Check sheet for the modelled part. Datum: model origin and axes. Units: mm. A direction names the side the tool comes from. Give positions to 0.01 mm unless a question says otherwise; leave off trailing zeros. Write each loop counter-clockwise with the first axis right and the second up, starting at its lowest first coordinate (ties: lowest second). Pieces come first, ordered by that corner, then holes. Notation, with made-up numbers: M 11,27 L 45,27 A25 ccw 45,58 Z; hole C 22.25,37 d8. An arc over 180 degrees is marked long. Write item = value, one per line. Start each with the question number.
1) Scan lines: L1, parallel to Y at x = 13.5, z = 0; L2, parallel to Y at x = 37.5, z = -59. Record each from-to range of solid material in increasing order.
2) Draft check along Z on faces 3 (the face through (1.97, 20.85, -32.11)), 4 (the face through (0, 0, 0)). Enter one of: pulls with the +Z half, pulls with the -Z half, needs draft (parallel to the pull), parting line crosses it, or undercut.
3) Gauge pin test, flat ends, axial feed: pin 1 (12 mm diameter, centred on x = 10, z = -8, fed in from -Y); pin 2 (10 mm diameter, centred on y = -2, z = 3.5, fed in from -X); pin 3 (2 mm diameter, centred on x = 6, y = 14, fed in from -Z); pin 4 (10 mm diameter, centred on y = -10, z = 39.5, fed in from +X). Record the tip position at first contact, or that the pin passes through.
4) Set-up check for faces 1 (the face through (1.97, 58.69, -33.34)), 2 (the face through (4, 0, 0)): record each of +Z, -Z, +X, -X, +Y, -Y from which the full face is reachable in a straight line by a thin tool's end or side.
5) Sectioned sample at C-C, the plane y = -43. Record the cut outline in (x, z), then the cut area to 3 significant figures.
6) Sectioned sample at D-D, the plane x = 34.5. Record the cut outline in (y, z), then the cut area to 3 significant figures.
7) Sectioned sample at B-B, the plane z = 48. Record the cut outline in (x, y).
8) Sectioned sample at A-A, the plane y = -22. Record the cut outline in (x, z).
Autodesk Inventor part; units mm, degrees
ref_plane "YZ Plane" through (0, 0, 0) normal (1, 0, 0) x (0, 1, 0)
ref_plane "XZ Plane" through (0, 0, 0) normal (0, 1, 0) x (-1, 0, 0)
ref_plane "XY Plane" through (0, 0, 0) normal (0, 0, 1) x (1, 0, 0)
sketch "Sketch1" plane through (0, 0, 0) normal (1, 0, 0) x (0, 1, 0)
  arc A0 (35.4672, -57.431) -> (67.4704, -2) centre (0, 0) ccw
  circle A1 centre (0, 0) radius 71.5
  arc A2 (3.1669, 9.4853) -> (-3.1669, 9.4853) centre (0, 0) ccw
  line L0 (10, 0) -> (67.5, 0) construction
  line L1 (9.798, 2) -> (67.4704, 2)
  line L2 (9.798, -2) -> (67.4704, -2)
  line L3 (3.1669, 9.4853) -> (32.0031, 59.431)
  line L4 (6.631, 7.4853) -> (35.4672, 57.431)
  line L5 (-6.631, 7.4853) -> (-35.4672, 57.431)
  line L6 (-3.1669, 9.4853) -> (-32.0031, 59.431)
  line L7 (-9.798, -2) -> (-67.4704, -2)
  line L8 (-9.798, 2) -> (-67.4704, 2)
  line L9 (-3.1669, -9.4853) -> (-32.0031, -59.431)
  line L10 (-6.631, -7.4853) -> (-35.4672, -57.431)
  line L11 (6.631, -7.4853) -> (35.4672, -57.431)
  line L12 (3.1669, -9.4853) -> (32.0031, -59.431)
  arc A3 (6.631, 7.4853) -> (3.1669, 9.4853) centre (0, 0) ccw
  arc A4 (-6.631, 7.4853) -> (-9.798, 2) centre (0, 0) ccw
  arc A5 (-3.1669, 9.4853) -> (-6.631, 7.4853) centre (0, 0) ccw
  arc A6 (-9.798, 2) -> (-9.798, -2) centre (0, 0) ccw
  arc A7 (-9.798, -2) -> (-6.631, -7.4853) centre (0, 0) ccw
  arc A8 (-6.631, -7.4853) -> (-3.1669, -9.4853) centre (0, 0) ccw
  arc A9 (-3.1669, -9.4853) -> (3.1669, -9.4853) centre (0, 0) ccw
  arc A10 (3.1669, -9.4853) -> (6.631, -7.4853) centre (0, 0) ccw
  arc A11 (6.631, -7.4853) -> (6.631, 7.4853) centre (0, 0) ccw
  arc A12 (32.0031, -59.431) -> (35.4672, -57.431) centre (0, 0) ccw
  arc A13 (67.4704, -2) -> (67.4704, 2) centre (0, 0) ccw construction
  arc A14 (35.4672, 57.431) -> (32.0031, 59.431) centre (0, 0) ccw construction
  arc A15 (32.0031, 59.431) -> (-32.0031, 59.431) centre (0, 0) ccw
  arc A16 (-32.0031, 59.431) -> (-35.4672, 57.431) centre (0, 0) ccw construction
  arc A17 (-35.4672, 57.431) -> (-67.4704, 2) centre (0, 0) ccw
  arc A18 (-67.4704, 2) -> (-67.4704, -2) centre (0, 0) ccw construction
  arc A19 (-67.4704, -2) -> (-35.4672, -57.431) centre (0, 0) ccw
  arc A20 (-35.4672, -57.431) -> (-32.0031, -59.431) centre (0, 0) ccw construction
  arc A21 (-32.0031, -59.431) -> (32.0031, -59.431) centre (0, 0) ccw
  arc A22 (67.4704, 2) -> (35.4672, 57.431) centre (0, 0) ccw
  dimension "d0" = 135
  dimension "d1" = 4
  dimension "d2" = 20
  dimension "d3" = 2
  dimension "d4" = 2
  dimension "d7" = 360
extrude "Extrusion1" add sketch "Sketch1" along normal blind 4 contours A12 L12 A10 L11 | A10 A9 A8 A7 A6 A4 A5 A2 A3 A11 | A1
sketch "Sketch2" plane through (4, 0, 0) normal (1, 0, 0) x (0, 0, -1)
  circle A0 centre (0, 0) radius 71.5
  line L0 (-59.431, 32.0031) -> (-9.4853, 3.1669)
  circle A1 centre (0, 0) radius 67.5
extrude "Extrusion2" add sketch "Sketch2" along normal blind 40
properties part number "SuportMotor"
Data:
q1.L1 = -71.5 to -67.5, 67.5 to 71.5
q1.L2 = -40.39 to -32.79, 32.79 to 40.39
q2.face_3 = undercut
q2.face_4 = needs draft
q3.pin_1 = -71.47
q3.pin_2 = 0
q3.pin_3 = -70.31
q3.pin_4 = through
q4.face_1 = +X, -X
q4.face_2 = +X
q5.outline = M 0,-57.12 L 44,-57.12 L 44,-52.03 L 0,-52.03 Z; M 0,-2 L 4,-2 L 4,2 L 0,2 Z; M 0,52.03 L 44,52.03 L 44,57.12 L 0,57.12 Z
q5.area = 464 mm2
q6.outline = C 0,0 d143; hole C 0,0 d135
q6.area = 1,750 mm2
q7.outline = M 0,-52.99 L 44,-52.99 L 44,-47.46 L 0,-47.46 Z; M 0,-30.02 L 4,-30.02 L 4,-25.4 L 0,-25.4 Z; M 0,25.4 L 4,25.4 L 4,30.02 L 0,30.02 Z; M 0,47.46 L 44,47.46 L 44,52.99 L 0,52.99 Z
q8.outline = M 0,-68.03 L 44,-68.03 L 44,-63.81 L 0,-63.81 Z; M 0,-42.11 L 4,-42.11 L 4,-34.11 L 0,-34.11 Z; M 0,-2 L 4,-2 L 4,2 L 0,2 Z; M 0,34.11 L 4,34.11 L 4,42.11 L 0,42.11 Z; M 0,63.81 L 44,63.81 L 44,68.03 L 0,68.03 Z
